Check sheet for the modelled part. Datum: model origin and axes. Units: mm. A direction names the side the tool comes from. Round coordinates to 2 decimals unless told otherwise and drop trailing zeros. Write each loop counter-clockwise with the first axis right and the second up, starting at its lowest first coordinate (ties: lowest second). Pieces come first, ordered by that corner, then holes.
from build123d import *

# Parameters (mm, degrees)
F1_W     = 101.6
F1_H     = 203.2
F2_DEPTH = 12.7
F3_W     = 152.4
F3_H     = 203.2
F4_DEPTH = 12.7
F6_D     = 14.2875
F6_DEPTH = 50.8
F6_TIP   = 4.2923980472
F8_DEPTH = 6.35


# Not quite as in the source:
# - a length typed as a fraction of an inch, garbled in the dataset ("3 / 203.2 mm" for 3/8 in), is restored


with BuildPart() as f2:
    # F1 (on offset) → F2 (new body)
    with BuildSketch(Plane.XY.offset(330.2)):
        Rectangle(F1_W, F1_H)
        with BuildLine():
            ThreePointArc((-38.1, -66.04), (-43.688, -60.452), (-38.1, -54.864))
            Line((-38.1, -54.864), (38.1, -54.864))
            ThreePointArc((38.1, -54.864), (43.688, -60.452), (38.1, -66.04))
            Line((38.1, -66.04), (-38.1, -66.04))
        make_face(mode=Mode.SUBTRACT)
        with BuildLine():
            Line((38.1, 54.864), (-38.1, 54.864))
            ThreePointArc((-38.1, 54.864), (-43.688, 60.452), (-38.1, 66.04))
            Line((-38.1, 66.04), (38.1, 66.04))
            ThreePointArc((38.1, 66.04), (43.688, 60.452), (38.1, 54.864))
        make_face(mode=Mode.SUBTRACT)
    extrude(amount=-F2_DEPTH)



with BuildPart() as f4:
    # F3 (on Top) → F4 (new body)
    with BuildSketch(Plane.XY):
        with Locations((50.8, 0)):
            Rectangle(F3_W, F3_H)
    extrude(amount=F4_DEPTH)

    # F6
    with Locations(Plane.XY.offset(12.7)):
        with Locations((0, 76.2), (101.6, 76.2), (0, -76.2), (101.6, -76.2)):
            Hole(F6_D / 2, depth=F6_DEPTH)
            with Locations((0, 0, -(F6_DEPTH + F6_TIP / 2))):  # 118° drill point
                Cone(0, F6_D / 2, F6_TIP, mode=Mode.SUBTRACT)


with BuildPart() as f2_1:
    add(f2.part)

    add(f4.part)  # F8 merges F4
    # F7 (on face) → F8 (join, symmetric)
    with BuildSketch(Plane.XZ.offset(101.6)):
        Polygon((50.8, 317.5), (-50.8, 317.5), (-25.4, 12.7), (127, 12.7), align=None)
    extrude(amount=F8_DEPTH, both=True)

    # F9: F2 across plane


with BuildPart() as f2_2:
    add(f2_1.part)
    add(f2_1.part.mirror(Plane.XZ))


solid = f2_2.part
1. Go/stop test with flat-tipped pins: pin 1 (3 mm diameter, centred on x = 62.5, y = -104, fed in from -Z); pin 2 (6.5 mm diameter, centred on x = -8, z = 322, fed in from -Y); pin 3 (10 mm diameter, centred on y = 46.5, z = 8.5, fed in from -X). Record where each tip stops, or that it passes through.
2. Sectioned sample at B-B, the plane y = -76.2. Enter the section's corners in (x, z).
3. Scan lines: line 1 along Y through (x, z) = (101.6, 10); line 2 along X through (y, z) = (76, 4); line 3 along Y through (x, z) = (3.5, 28.5). Record each from-to range of solid material in increasing order.
4. Sectioned sample at A-A, the plane x = 101.6. Enter the section's corners in (y, z), plus the area to 3 significant figures.
5. Sectioned sample at C-C, the plane x = -21.5. Enter the section's corners in (y, z).
6. Sectioned sample at D-D, the plane z = 170.5. Enter the section's corners in (x, y), plus the area to 3 significant figures.
7. Set-up check for faces 1 (the flat face through (17, -95.25, 167)), 2 (the flat face through (50.8, -1, 324)), 3 (the flat face through (-1, 66.04, 324)), 4 (the cylindrical face through (-43.687, -60.575, 323.939)), 5 (the flat face through (50, 1, 0)): record each of +Z, -Z, +X, -X, +Y, -Y from which the full face is reachable in a straight line by a thin tool's end or side.
8. Release check for a two-part mould opening along X. For faces 6 (the flat face through (-1, 101.6, 324)), 7 (the cylindrical face through (-43.687, 60.329, 323.939)), 8 (the flat face through (-38.278, -101.689, 167.234)), 9 (the cylindrical face through (0.93, -69.117, 6.261)) record: released by +X, released by -X, zero draft, split by the parting line, or undercut.
Computed values:
1. pin 1: stops at z = 12.7
1. pin 2: stops at y = -101.6
1. pin 3: stops at x = -25.4
2. outline: (-50.8, 317.5) - (50.8, 317.5) - (50.8, 330.2) - (-50.8, 330.2) - close; (-25.4, 0) - (-7.14, 0) - (-7.14, 12.7) - (-25.4, 12.7) - close; (7.14, 0) - (94.46, 0) - (94.46, 12.7) - (7.14, 12.7) - close; (108.74, 0) - (127, 0) - (127, 12.7) - (108.74, 12.7) - close
3. line 1: y = -101.6 to -83.34, -69.06 to 69.06, 83.34 to 101.6
3. line 2: x = -25.4 to -7.14, 7.14 to 94.46, 108.74 to 127
3. line 3: y = -107.95 to -95.25, 95.25 to 107.95
4. outline: (-107.95, 12.7) - (-101.6, 12.7) - (-101.6, 0) - (-83.34, 0) - (-83.34, 12.7) - (-95.25, 12.7) - (-95.25, 114.3) - (-107.95, 114.3) - close; (-69.06, 0) - (69.06, 0) - (69.06, 12.7) - (-69.06, 12.7) - close; (83.34, 0) - (101.6, 0) - (101.6, 12.7) - (107.95, 12.7) - (107.95, 114.3) - (95.25, 114.3) - (95.25, 12.7) - (83.34, 12.7) - close
4. area: 4,800 mm2
5. outline: (-107.95, 12.7) - (-101.6, 12.7) - (-101.6, 0) - (101.6, 0) - (101.6, 12.7) - (107.95, 12.7) - (107.95, 317.5) - (101.6, 317.5) - (101.6, 330.2) - (66.04, 330.2) - (66.04, 317.5) - (95.25, 317.5) - (95.25, 12.7) - (-95.25, 12.7) - (-95.25, 317.5) - (-66.04, 317.5) - (-66.04, 330.2) - (-101.6, 330.2) - (-101.6, 317.5) - (-107.95, 317.5) - close; (-54.86, 317.5) - (54.86, 317.5) - (54.86, 330.2) - (-54.86, 330.2) - close
6. outline: (-38.55, -107.95) - (87.55, -107.95) - (87.55, -95.25) - (-38.55, -95.25) - close; (-38.55, 95.25) - (87.55, 95.25) - (87.55, 107.95) - (-38.55, 107.95) - close
6. area: 3,200 mm2
7. face 1: +X, -X
7. face 2: +Z, +X, +Y, -Y
7. face 3: +Z
7. face 4: +Z, -Z
7. face 5: -Z, +X, -X, +Y, -Y
8. face 6: zero draft
8. face 7: undercut
8. face 8: released by -X
8. face 9: undercut
